from build123d import *
from OCP.BRepFilletAPI import BRepFilletAPI_MakeChamfer

# Parameters (mm, degrees)
SKETCH1_W               = 8
SKETCH1_H               = 3.8
BOSS_EXTRUDE1_DEPTH     = 2.5
CHAMFER1_SIZE           = 1.5
CHAMFER1_SIZE2          = 0.401923789
CHAMFER2_SIZE           = 1.5
CHAMFER2_SIZE2          = 1.060660172
SKETCH2_W               = 0.5
SKETCH2_H               = 0.1
LPATTERN1_COUNT         = 2
LPATTERN1_PITCH         = 5.5
MIRROR1_COPY_1_SKETCH_W = 0.5
MIRROR1_COPY_1_SKETCH_H = 0.1


with BuildPart() as part:
    # Sketch1 → Boss-Extrude1 (new body)
    with BuildSketch(Plane(origin=(0, 0, 0), x_dir=(1, 0, 0), z_dir=(0, 1, 0))):
        Rectangle(SKETCH1_W, SKETCH1_H)
    extrude(amount=BOSS_EXTRUDE1_DEPTH)

    # Chamfer1: one chamfer whose edges measure the first distance from different faces: ONE call of the kernel's chamfer builder (chamfer() names one face for all edges)
    chamfer1_edges_1 = [part.edges().sort_by_distance(p)[0] for p in [
        (-4, 2.5, 0),
    ]]
    chamfer1_side_1 = [part.faces().sort_by_distance(p)[0] for p in [
        (-4, 1.25, 0),
    ]]
    chamfer1_edges_2 = [part.edges().sort_by_distance(p)[0] for p in [
        (0, 2.5, 1.9),
    ]]
    chamfer1_side_2 = [part.faces().sort_by_distance(p)[0] for p in [
        (0, 1.25, 1.9),
    ]]
    chamfer1_edges_3 = [part.edges().sort_by_distance(p)[0] for p in [
        (4, 2.5, 0),
    ]]
    chamfer1_side_3 = [part.faces().sort_by_distance(p)[0] for p in [
        (4, 1.25, 0),
    ]]
    chamfer1_edges_4 = [part.edges().sort_by_distance(p)[0] for p in [
        (0, 2.5, -1.9),
    ]]
    chamfer1_side_4 = [part.faces().sort_by_distance(p)[0] for p in [
        (0, 1.25, -1.9),
    ]]
    chamfer1 = BRepFilletAPI_MakeChamfer(part.part.solid().wrapped)
    for e in chamfer1_edges_1:
        chamfer1.Add(CHAMFER1_SIZE, CHAMFER1_SIZE2, e.wrapped, chamfer1_side_1[0].wrapped)  # the first distance lies on this face
    for e in chamfer1_edges_2:
        chamfer1.Add(CHAMFER1_SIZE, CHAMFER1_SIZE2, e.wrapped, chamfer1_side_2[0].wrapped)  # the first distance lies on this face
    for e in chamfer1_edges_3:
        chamfer1.Add(CHAMFER1_SIZE, CHAMFER1_SIZE2, e.wrapped, chamfer1_side_3[0].wrapped)  # the first distance lies on this face
    for e in chamfer1_edges_4:
        chamfer1.Add(CHAMFER1_SIZE, CHAMFER1_SIZE2, e.wrapped, chamfer1_side_4[0].wrapped)  # the first distance lies on this face
    add(Compound.cast(chamfer1.Shape()), mode=Mode.REPLACE)

    # Chamfer2
    chamfer2_edges = [part.edges().sort_by_distance(p)[0] for p in [
        (-3.598076211, 2.5, 0),
    ]]
    chamfer2_side = [part.faces().sort_by_distance(p)[0] for p in [
        (-3.80696135, 1.720430049, 0),
    ]]
    chamfer(chamfer2_edges, length=CHAMFER2_SIZE, length2=CHAMFER2_SIZE2, reference=chamfer2_side[0])

    # Sweep1: sweep along a path in Sketch3
    with BuildLine(Plane(origin=(-2.75, 0, 0), x_dir=(0, 0, -1), z_dir=(1, 0, 0))) as sweep1_path:
        Line((-1.9, 0.949951684), (-2.05, 0.949951684))
        Line((-2.05, 0.949951684), (-2.05, -0.150048316))
        Line((-2.05, -0.150048316), (-1.162596201, 0))
    # Sketch2 → Sweep1 (sweep)
    with BuildSketch(Plane.XY.offset(1.9)):
        with Locations((-2.75, 0.949951684)):
            Rectangle(SKETCH2_W, SKETCH2_H)
    sweep1 = sweep(path=sweep1_path.line, transition=Transition.RIGHT)

    # LPattern1: Sweep1 ×2
    with Locations(*[(i * LPATTERN1_PITCH, 0, 0) for i in range(1, LPATTERN1_COUNT)]):
        add(sweep1)

    # Mirror1: Sweep1 across plane
    add(sweep1.mirror(Plane.XY))

    # Mirror1 copy 1: sweep along a path in Mirror1 copy 1 path
    with BuildLine(Plane(origin=(2.75, 0, 0), x_dir=(0, 0, 1), z_dir=(1, 0, 0))) as mirror1_copy_1_path:
        Line((-1.9, -0.949951684), (-2.05, -0.949951684))
        Line((-2.05, -0.949951684), (-2.05, 0.150048316))
        Line((-2.05, 0.150048316), (-1.162596201, 0))
    # Mirror1 copy 1 sketch → Mirror1 copy 1 (sweep)
    with BuildSketch(Plane(origin=(5.5, 0, -1.9), x_dir=(1, 0, 0), z_dir=(0, 0, -1))):
        with Locations((-2.75, -0.949951684)):
            Rectangle(MIRROR1_COPY_1_SKETCH_W, MIRROR1_COPY_1_SKETCH_H)
    sweep(path=mirror1_copy_1_path.line, transition=Transition.RIGHT)


solid = part.part
Source: CAD feature listing. Evaluate the final solid. Frame: model axes, mm. Coordinates: 2 decimals unless noted, no trailing zeros. Loops run counter-clockwise (first coordinate to the right, second up) from the corner with the lowest first, then second, coordinate; pieces in that order, holes last. Notation, with made-up numbers: (78, 62) -> (132, 62) arc R31 cw to (132, 92) -> close; hole circle Ø6 at (71.25, -2.5). An arc over 180 degrees is marked (long way). Answer in a Markdown table with one row per item. Add a question column.
Q1. Section B-B on z = 1.75. Return the cut outline in (x, y), and give its area (3 significant figures).
Q2. Section A-A on y = 0.25. Return the cut outline in (x, z).
Q3. Section C-C on x = -0.5. Return the cut outline in (y, z), and give its area (3 significant figures).
Q4. Ray query, line 1 along Y through (x, z) = (1.5, 0.7); line 2 along Z through (x, y) = (-0.75, 0.15); line 3 along X through (y, z) = (1.6, -1.05). Return the intervals inside material, ascending.
Q5. Section D-D on z = 0.9. Return the cut outline in (x, y), and give its area (3 significant figures).
Q6. Contact query for flat-ended pins moving along their axis: pin 1 Ø0.5 at (x, y) = (1, 0.5) entering from -Z; pin 2 Ø1.5 at (x, y) = (-1, 1) entering from +Z. Output: stop coordinate, or through.
Computed values:
| question | item | result |
|---|---|---|
| 1 | outline | (-4, 0) -> (4, 0) -> (4, 1) -> (3.85, 1.56) -> (-3.48, 1.56) -> (-3.99, 1.05) -> (-4, 1) -> close; (-3, -0.15) -> (-2.5, -0.15) -> (-2.5, -0.05) -> (-3, -0.05) -> close; (2.5, -0.15) -> (3, -0.15) -> (3, -0.05) -> (2.5, -0.05) -> close |
| 1 | area | 12.4 mm^2 |
| 2 | outline | (-4, -1.9) -> (4, -1.9) -> (4, 1.9) -> (-4, 1.9) -> close; (-3, -2.1) -> (-2.5, -2.1) -> (-2.5, -2) -> (-3, -2) -> close; (-3, 2) -> (-2.5, 2) -> (-2.5, 2.1) -> (-3, 2.1) -> close; (2.5, -2.1) -> (3, -2.1) -> (3, -2) -> (2.5, -2) -> close; (2.5, 2) -> (3, 2) -> (3, 2.1) -> (2.5, 2.1) -> close |
| 3 | outline | (0, -1.9) -> (1, -1.9) -> (2.5, -1.5) -> (2.5, 1.5) -> (1, 1.9) -> (0, 1.9) -> close |
| 3 | area | 8.90 mm^2 |
| 4 | line 1 | y = 0 to 2.5 |
| 4 | line 2 | z = -1.9 to 1.9 |
| 4 | line 3 | x = -3.44 to 3.84 |
| 5 | outline | (-4, 0) -> (4, 0) -> (4, 1) -> (3.6, 2.5) -> (-2.54, 2.5) -> (-3.99, 1.05) -> (-4, 1) -> close |
| 5 | area | 18.6 mm^2 |
| 6 | pin 1 | stops at z = -1.9 |
| 6 | pin 2 | stops at z = 1.9 |
